Work out the finished part from the listing and answer in its coordinate system (mm). Face numbers are marked on the shaded views. A direction names the side the tool comes from. Give positions to 0.01 mm unless a question says otherwise; leave off trailing zeros. Write each loop counter-clockwise with the first axis right and the second up, starting at its lowest first coordinate (ties: lowest second). Pieces come first, ordered by that corner, then holes.
1) A tool of negligible diameter and unlimited length cuts with its end or side. For the marked faces 4, 5 and 6, from which of +Z, -Z, +X, -X, +Y, -Y can it reach the whole face along a straight path? Write none if from no direction.
2) Find section A-A (y = 44.5). Determine the outline of the cut face in (x, z), plus the area to 3 significant figures.
3) Straight lines are drawn through the part: probe 1 along Z at (x, y) = (241.3, 70.5); probe 2 along X at (y, z) = (44.5, 19); probe 3 along Y at (x, z) = (226, 3.75). For each, find the intervals that lie inside material, in ascending order.
4) Find section C-C (x = 368.3). Determine the outline of the cut face in (y, z) (3 decimals).
5) Given pin 1 Ø5.5 at (x, z) = (215.9, 12.7) entering from -Y; pin 2 Ø2 at (y, z) = (32.5, 18) entering from -X, each flat-ended and moving along its own axis, determine where each tip first touches the part or whether it passes through.
6) Find section B-B (x = 197). Determine the outline of the cut face in (y, z), plus the area to 3 significant figures.
7) Determine the mould class of the marked faces 1, 2 and 3 for opening direction Y: pulls with the +Y half, pulls with the -Y half, needs draft (parallel to the pull), parting line crosses it, or undercut.
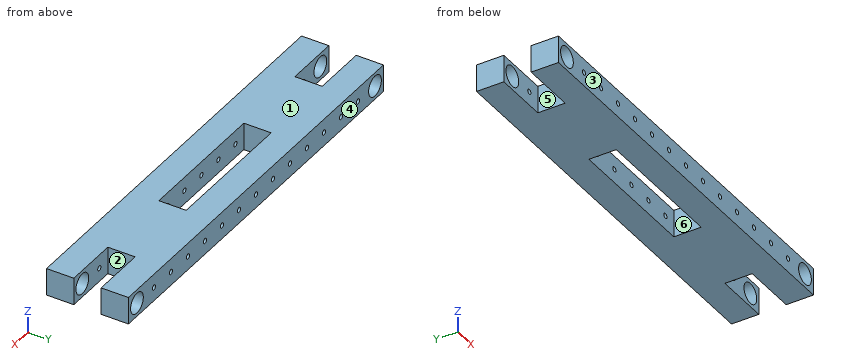
Autodesk Inventor part; units mm, degrees
ref_plane "YZ Plane" through (0, 0, 0) normal (1, 0, 0) x (0, 1, 0)
ref_plane "XZ Plane" through (0, 0, 0) normal (0, 1, 0) x (-1, 0, 0)
ref_plane "XY Plane" through (0, 0, 0) normal (0, 0, 1) x (1, 0, 0)
sketch "Sketch1" plane through (0, 0, 0) normal (0, 0, 1) x (1, 0, 0)
  line L0 (0, 0) -> (381, 0)
  line L1 (381, 0) -> (381, 76.2)
  line L2 (381, 76.2) -> (0, 76.2)
  line L3 (0, 76.2) -> (0, 0)
  dimension "d0" = 381
  dimension "d1" = 76.2
extrude "Extrusion1" add sketch "Sketch1" along normal blind 25.4
sketch "Sketch7" plane through (0, 0, 25.4) normal (0, 0, 1) x (1, 0, 0)
  line L0 (0, 50.8) -> (50.8, 50.8)
  line L1 (50.8, 50.8) -> (50.8, 25.4)
  line L2 (50.8, 25.4) -> (0, 25.4)
  line L3 (0, 25.4) -> (0, 50.8)
  line L4 (127, 50.8) -> (254, 50.8)
  line L5 (254, 50.8) -> (254, 25.4)
  line L6 (254, 25.4) -> (127, 25.4)
  line L7 (127, 25.4) -> (127, 50.8)
  line L8 (330.2, 50.8) -> (381, 50.8)
  line L9 (381, 50.8) -> (381, 25.4)
  line L10 (381, 25.4) -> (330.2, 25.4)
  line L11 (330.2, 25.4) -> (330.2, 50.8)
  line L12 (381, 76.2) -> (0, 76.2)
  line L13 (0, 0) -> (381, 0)
  line L14 (0, 76.2) -> (0, 0)
  line L15 (381, 0) -> (381, 76.2)
  dimension "d34" = 25.4
  dimension "d35" = 25.4
  dimension "d36" = 25.4
  dimension "d37" = 25.4
  dimension "d38" = 0
  dimension "d39" = 0
  dimension "d40" = 76.2
  dimension "d41" = 76.2
  dimension "d42" = 50.8
  dimension "d43" = 50.8
extrude "Extrusion6" cut sketch "Sketch7" against normal blind 25.4 contours L0 L1 L2 L3 | L9 L10 L11 L8 | L4 L5 L6 L7
sketch "Sketch8" plane through (0, 76.2, 0) normal (0, 1, 0) x (1, 0, 0)
  circle A0 centre (12.7, -12.7) radius 2.3812
  line L0 (381, -25.4) -> (0, -25.4)
  circle A1 centre (38.1, -12.7) radius 2.3812
  circle A2 centre (63.5, -12.7) radius 2.3812
  circle A3 centre (88.9, -12.7) radius 2.3812
  circle A4 centre (114.3, -12.7) radius 2.3812
  circle A5 centre (139.7, -12.7) radius 2.3812
  circle A6 centre (165.1, -12.7) radius 2.3812
  circle A7 centre (190.5, -12.7) radius 2.3812
  circle A8 centre (215.9, -12.7) radius 2.3812
  circle A9 centre (241.3, -12.7) radius 2.3812
  circle A10 centre (266.7, -12.7) radius 2.3812
  circle A11 centre (292.1, -12.7) radius 2.3812
  circle A12 centre (317.5, -12.7) radius 2.3812
  line L1 (0, 0) -> (0, -25.4)
  circle A13 centre (342.9, -12.7) radius 2.3812
  circle A14 centre (368.3, -12.7) radius 2.3812
  circle A15 centre (368.3, -12.7) radius 9.525
  circle A16 centre (12.7, -12.7) radius 9.525
  dimension "d46" = 4.7625
  dimension "d47" = 12.7
  dimension "d50" = 25.4
  dimension "d55" = 12.7
  dimension "d58" = 19.05
  dimension "d59" = 19.05
extrude "Extrusion7" cut sketch "Sketch8" against normal blind 76.2 contours A0 | A1 | A2 | A3 | A4 | A5 | A6 | A7 | A8 | A9 | A10 | A11 | A12 | A13 | A14 | A15 | A16
equation "\"d35\" = d34"
equation "\"d37\" = d36"
properties part number "RobotArm Board"
Results:
1. face 4: +Z, -Z, +X, -X, +Y
1. face 5: +Z, -Z, -X
1. face 6: +Z, -Z
2. outline: (50.8, 0) - (127, 0) - (127, 25.4) - (50.8, 25.4) - close; (254, 0) - (330.2, 0) - (330.2, 25.4) - (254, 25.4) - close; hole circle Ø4.76 at (63.5, 12.7); hole circle Ø4.76 at (88.9, 12.7); hole circle Ø4.76 at (114.3, 12.7); hole circle Ø4.76 at (266.7, 12.7); hole circle Ø4.76 at (292.1, 12.7); hole circle Ø4.76 at (317.5, 12.7)
2. area: 3,760 mm2
3. probe 1: z = 0 to 10.32, 15.08 to 25.4
3. probe 2: x = 50.8 to 127, 254 to 330.2
3. probe 3: y = 0 to 25.4, 50.8 to 76.2
4. outline: (0, 0) - (25.4, 0) - (25.4, 3.175) - (0, 3.175) - close; (0, 22.225) - (25.4, 22.225) - (25.4, 25.4) - (0, 25.4) - close; (50.8, 0) - (76.2, 0) - (76.2, 3.175) - (50.8, 3.175) - close; (50.8, 22.225) - (76.2, 22.225) - (76.2, 25.4) - (50.8, 25.4) - close
5. pin 1: stops at y = 0
5. pin 2: stops at x = 50.8
6. outline: (0, 0) - (25.4, 0) - (25.4, 25.4) - (0, 25.4) - close; (50.8, 0) - (76.2, 0) - (76.2, 25.4) - (50.8, 25.4) - close
6. area: 1,290 mm2
7. face 1: needs draft
7. face 2: undercut
7. face 3: pulls with the -Y half
